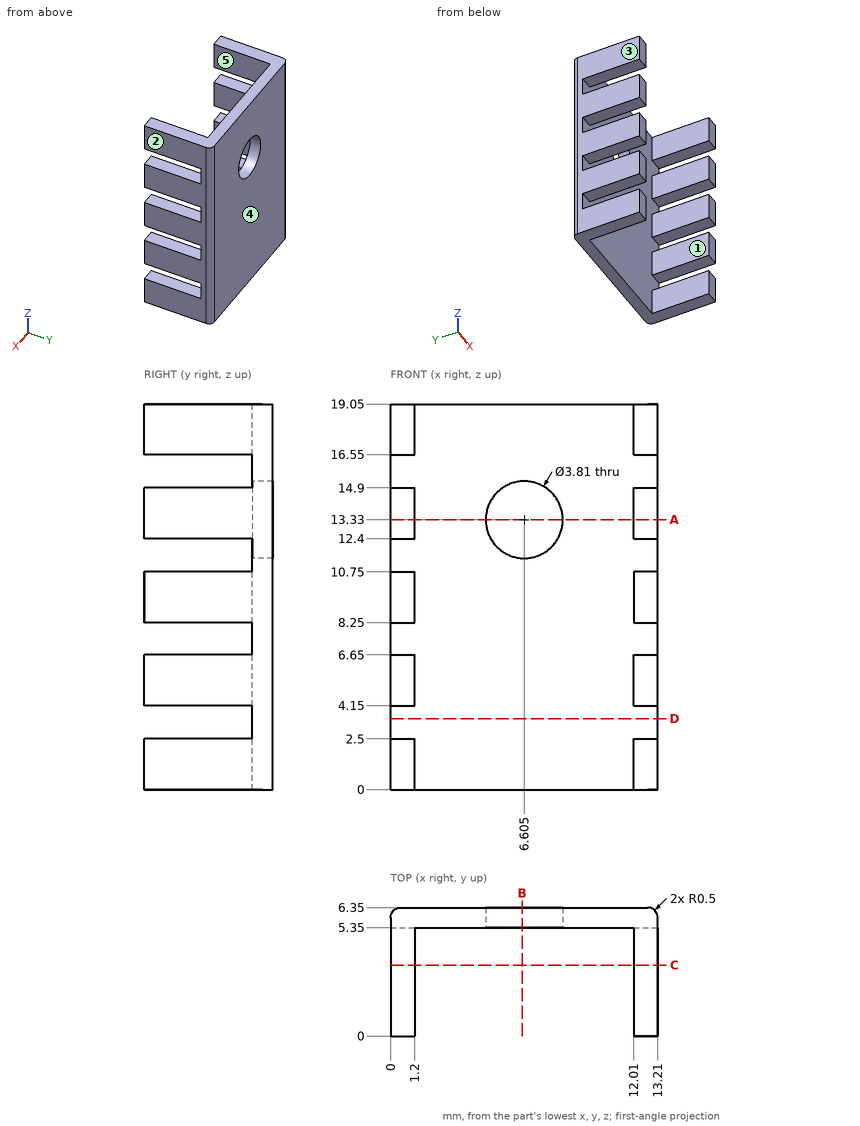
The figure shows three views and two pictorial views of one solid part (mm, origin at its lowest corner). Answer the questions. A direction names the side the tool comes from. Round coordinates to 2 decimals unless told otherwise and drop trailing zeros. Write each loop counter-clockwise with the first axis right and the second up, starting at its lowest first coordinate (ties: lowest second). Pieces come first, ordered by that corner, then holes. Notation, with made-up numbers: (-10, -24.5) - (34, -24.5) arc R36 ccw to (34, 13.5) - close; hole circle Ø8 at (72, 62.5). An arc over 180 degrees is marked (long way). Use one line per item in the form item = value. Start each with the question number.
Item 1: A cutting plane is placed at D-D (z = 3.5). Write down the section's boundary in (x, y), plus the area to 3 significant figures.
Item 2: Determine the mould class of the marked faces 3, 4 and 5 for opening direction X: +X half, -X half, draft (parallel to the pull), parting line (faces both ways), or undercut.
Item 3: Find the intervals of material crossed by line 1 (X direction, y = 5.25, z = 13.75); line 2 (Y direction, x = 6.75, z = 1.5); line 3 (X direction, y = 6, z = 2.5), in increasing order. Write a range as [from, to].
Item 4: A cutting plane is placed at A-A (z = 13.33). Write down the section's boundary in (x, y), plus the area to 3 significant figures.
Item 5: A tool of negligible diameter and unlimited length cuts with its end or side. For the marked faces 1 and 2, from which of +Z, -Z, +X, -X, +Y, -Y can it reach the whole face along a straight path? Write none if from no direction.
Item 6: A flat-ended cylindrical pin translates along its axis: pin 1 Ø5 at (x, z) = (9.5, 12) entering from -Y. Find the tip coordinate at first contact, or state that the pin passes through.
Item 7: A cutting plane is placed at C-C (y = 3.5). Give the number of separate pieces and of enclosed holes in the cut face, plus the area to 3 significant figures.
Item 8: A cutting plane is placed at B-B (x = 6.5). Write down the section's boundary in (y, z).
The answers:
q1.outline = (0, 5.35) - (13.21, 5.35) - (13.21, 5.85) arc R0.5 ccw to (12.71, 6.35) - (0.5, 6.35) arc R0.5 ccw to (0, 5.85) - close
q1.area = 13.1 mm^2
q2.face_3 = -X half
q2.face_4 = draft
q2.face_5 = undercut
q3.line_1 = [0, 1.2], [12.01, 13.21]
q3.line_2 = [5.35, 6.35]
q3.line_3 = [0.02, 13.19]
q4.outline = (0, 0) - (1.2, 0) - (1.2, 5.35) - (4.7, 5.35) - (4.7, 6.35) - (0.5, 6.35) arc R0.5 ccw to (0, 5.85) - close; (8.51, 5.35) - (12.01, 5.35) - (12.01, 0) - (13.21, 0) - (13.21, 5.85) arc R0.5 ccw to (12.71, 6.35) - (8.51, 6.35) - close
q4.area = 22.1 mm^2
q5.face_1 = +Z, -Z, -Y
q5.face_2 = +Z, -Z, +X, +Y, -Y
q6.pin_1 = 5.35
q7.separate_pieces = 10
q7.enclosed_holes = 0
q7.area = 30.0 mm^2
q8.outline = (5.35, 0) - (6.35, 0) - (6.35, 11.43) - (5.35, 11.43) - close; (5.35, 15.23) - (6.35, 15.23) - (6.35, 19.05) - (5.35, 19.05) - close
